Here's the drawing with two shaded views (mm, measured from the low corner). I have some questions. A direction names the side the tool comes from. Coordinates: 2 decimals unless noted, no trailing zeros. Write each loop counter-clockwise with the first axis right and the second up, starting at its lowest first coordinate (ties: lowest second). Pieces come first, ordered by that corner, then holes.
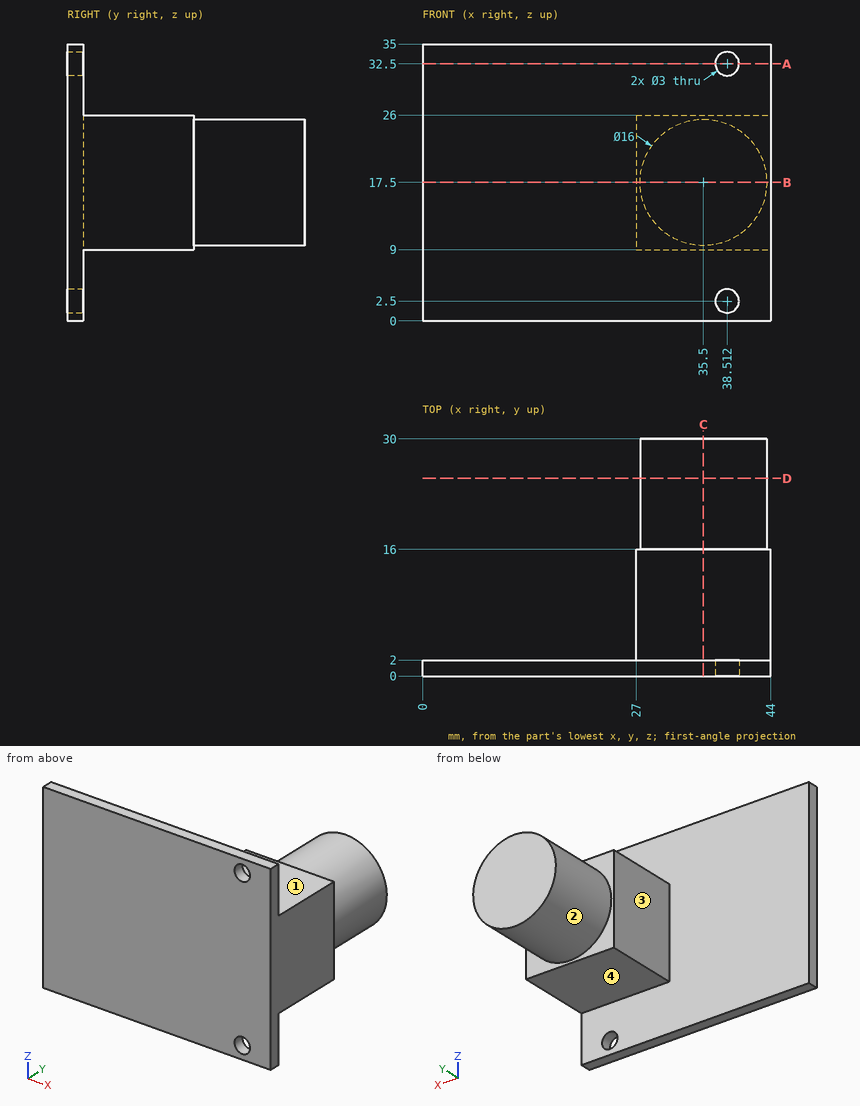
1. If I drill on L1, parallel to X at y = 1.4, z = 32.5; L2, parallel to Y at x = 15, z = 25; L3, parallel to Z at x = 29.5, y = 13.25, over which ranges is the centre line in solid material (lowest first)?
2. I'm going to push flat-ended pins straight in: P1, Ø15.5, axis at y = 11.5, z = 20, coming from the -X side; P2, Ø8, axis at y = 26.5, z = 11, coming from the +X side; P3, Ø11, axis at x = 35, y = 11, coming from the -Z side. Where does each tip first touch, or does it pass through?
3. If we section it at D-D, the plane y = 25: List the corners of the cut face in (x, z) for me, plus the area to 3 significant figures.
4. Which directions (+Z, -Z, +X, -X, +Y, -Y) give clear straight access to the entire face, cutting with the end or side of a thin tool? Please do the marked faces 1, 2, 3 and 4.
5. If we section it at B-B, the plane z = 17.5: List the corners of the cut face in (x, y) for me, plus the area to 3 significant figures.
6. If we section it at C-C, the plane x = 35.5: List the corners of the cut face in (y, z) for me.
7. If we section it at A-A, the plane z = 32.5: List the corners of the cut face in (x, y) for me.
Answers:
1. L1: x = 0 to 37.01, 40.01 to 44
1. L2: y = 0 to 2
1. L3: z = 9 to 26
2. P1: stops at x = 27
2. P2: stops at x = 43.1
2. P3: stops at z = 9
3. outline: circle Ø16 at (35.5, 17.5)
3. area: 201 mm2
4. face 1: +Z, +X, -X, +Y
4. face 2: +Y
4. face 3: +Z, -Z, -X, +Y
4. face 4: -Z, +X, -X, +Y
5. outline: (0, 0) - (44, 0) - (44, 16) - (43.5, 16) - (43.5, 30) - (27.5, 30) - (27.5, 16) - (27, 16) - (27, 2) - (0, 2) - close
5. area: 550 mm2
6. outline: (0, 0) - (2, 0) - (2, 9) - (16, 9) - (16, 9.5) - (30, 9.5) - (30, 25.5) - (16, 25.5) - (16, 26) - (2, 26) - (2, 35) - (0, 35) - close
7. outline: (0, 0) - (37.01, 0) - (37.01, 2) - (0, 2) - close; (40.01, 0) - (44, 0) - (44, 2) - (40.01, 2) - close
